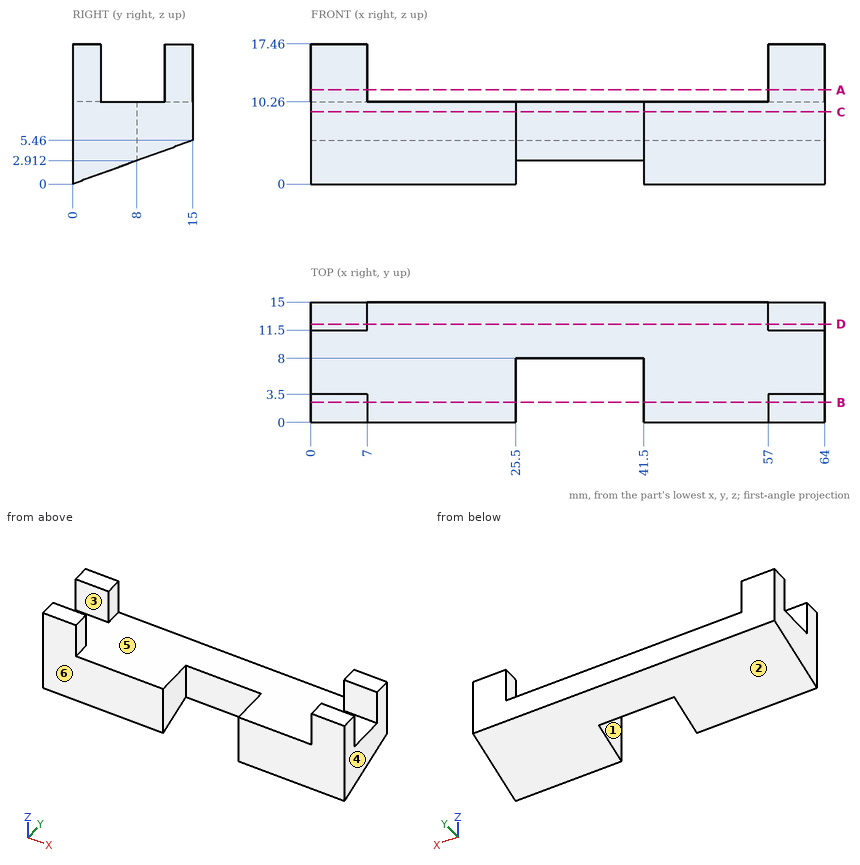
Design review of the part shown in the three views and the two pictorial views. Dimensions are in mm from the part's minimum x, y and z. A direction names the side the tool comes from. Coordinates: 2 decimals unless noted, no trailing zeros. Order: outer loops, then holes, each group sorted by start corner. A loop starts at its lowest first (then second) coordinate and runs counter-clockwise, first axis right, second up.
1) Take a section at D-D, the plane y = 12.25. Give the boundary of the cut face in (x, z), and give its area (3 significant figures).
2) For the marked faces 1, 2 and 3, list the 3-axis set-ups (+Z, -Z, +X, -X, +Y, -Y) from which the entire face can be reached by the end or side of a thin tool; tool diameter is ignored.
3) Take a section at C-C, the plane z = 9. Give the boundary of the cut face in (x, y).
4) Take a section at B-B, the plane y = 2.5. Give the boundary of the cut face in (x, z).
5) Clearance check with flat-ended pins moving along their axes: pin 1 (3 mm diameter, centred on x = 49, y = 6, fed in from +Z); pin 2 (6 mm diameter, centred on x = 35.5, z = 5, fed in from -Y). State where each tip first meets the part, or that it passes through.
6) Mouldability with a two-part tool opening along X and no side actions: class the marked faces 4, 5 and 6 as +X half, -X half, draft (parallel to the pull), parting line (faces both ways), or undercut.
7) Wall thickness on line 1 along X through (y, z) = (3, 6.5); line 2 along X through (y, z) = (1, 15.75); line 3 along Y through (x, z) = (33.5, 8.25): over which ranges is each line inside the solid? List them lowest first.
8) Take a section at A-A, the plane z = 11.75. Give the boundary of the cut face in (x, y).
Returned:
1. outline: (0, 4.46) - (64, 4.46) - (64, 17.46) - (57, 17.46) - (57, 10.26) - (7, 10.26) - (7, 17.46) - (0, 17.46) - close
1. area: 472 mm2
2. face 1: +Z, -Z, -Y
2. face 2: -Z, +X, -X, +Y
2. face 3: +Z, +X, -X
3. outline: (0, 0) - (25.5, 0) - (25.5, 8) - (41.5, 8) - (41.5, 0) - (64, 0) - (64, 15) - (0, 15) - close
4. outline: (0, 0.91) - (25.5, 0.91) - (25.5, 10.26) - (7, 10.26) - (7, 17.46) - (0, 17.46) - close; (41.5, 0.91) - (64, 0.91) - (64, 17.46) - (57, 17.46) - (57, 10.26) - (41.5, 10.26) - close
5. pin 1: stops at z = 10.26
5. pin 2: stops at y = 8
6. face 4: +X half
6. face 5: undercut
6. face 6: draft
7. line 1: x = 0 to 25.5, 41.5 to 64
7. line 2: x = 0 to 7, 57 to 64
7. line 3: y = 8 to 15
8. outline: (0, 0) - (7, 0) - (7, 3.5) - (0, 3.5) - close; (0, 11.5) - (7, 11.5) - (7, 15) - (0, 15) - close; (57, 0) - (64, 0) - (64, 3.5) - (57, 3.5) - close; (57, 11.5) - (64, 11.5) - (64, 15) - (57, 15) - close
